Read the model definition and answer for the solid it produces. Units are mm, in the model's axes. Face numbers are marked on the shaded views. A direction names the side the tool comes from. Round coordinates to 2 decimals unless told otherwise and drop trailing zeros. Write each loop counter-clockwise with the first axis right and the second up, starting at its lowest first coordinate (ties: lowest second). Pieces come first, ordered by that corner, then holes. Notation, with made-up numbers: (79.5, 27) -> (99.5, 27) arc R8 cw to (99.5, 34) -> close; hole circle Ø6 at (88, 46.25). An arc over 180 degrees is marked (long way). Return JSON: item names as keys, results as strings.
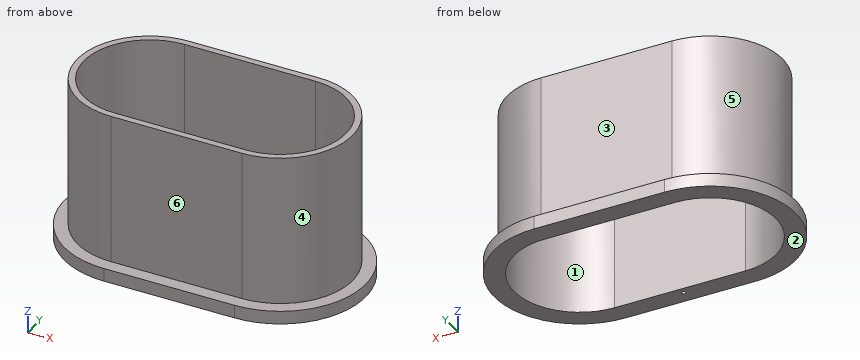
from build123d import *

# Parameters (mm, degrees)
EXTRUDE_1_DEPTH     = 2
EXTRUDE_2_DEPTH     = 23
SKETCH_4_R          = 0.3
CUT_EXTRUDE_2_DEPTH = 0.5


with BuildPart() as part:
    # 草图1 → 凸台-拉伸1 (new body)
    with BuildSketch(Plane.XY):
        with BuildLine():
            Line((-7.168044136, -16.461643491), (-27.168044136, -16.461643491))
            ThreePointArc((-27.168044136, -16.461643491), (-40.168044136, -3.461643491), (-27.168044136, 9.538356509))
            Line((-27.168044136, 9.538356509), (-7.168044136, 9.538356509))
            ThreePointArc((-7.168044136, 9.538356509), (5.831955864, -3.461643491), (-7.168044136, -16.461643491))
        make_face()
        with BuildLine():
            Line((-27.168044136, -13.461643491), (-7.168044136, -13.461643491))
            ThreePointArc((-7.168044136, -13.461643491), (2.831955864, -3.461643491), (-7.168044136, 6.538356509))
            Line((-7.168044136, 6.538356509), (-27.168044136, 6.538356509))
            ThreePointArc((-27.168044136, 6.538356509), (-37.168044136, -3.461643491), (-27.168044136, -13.461643491))
        make_face(mode=Mode.SUBTRACT)
    extrude(amount=EXTRUDE_1_DEPTH)

    # 草图2 → 凸台-拉伸2 (add)
    with BuildSketch(Plane.XY.offset(2)):
        with BuildLine():
            Line((-27.168044136, 7.538356509), (-7.168044136, 7.538356509))
            ThreePointArc((-7.168044136, 7.538356509), (3.831955864, -3.461643491), (-7.168044136, -14.461643491))
            Line((-7.168044136, -14.461643491), (-27.168044136, -14.461643491))
            ThreePointArc((-27.168044136, -14.461643491), (-38.168044136, -3.461643491), (-27.168044136, 7.538356509))
        make_face()
        with BuildLine():
            Line((-27.168044136, 6.538356509), (-7.168044136, 6.538356509))
            ThreePointArc((-7.168044136, 6.538356509), (2.831955864, -3.461643491), (-7.168044136, -13.461643491))
            Line((-7.168044136, -13.461643491), (-27.168044136, -13.461643491))
            ThreePointArc((-27.168044136, -13.461643491), (-37.168044136, -3.461643491), (-27.168044136, 6.538356509))
        make_face(mode=Mode.SUBTRACT)
    extrude(amount=EXTRUDE_2_DEPTH)

    # 草图4 → 切除-拉伸2 (cut)
    with BuildSketch(Plane(origin=(0, 0, 0), x_dir=(-1, 0, 0), z_dir=(0, 0, -1))):
        with Locations((17.168044136, -14.461643491)):
            Circle(SKETCH_4_R)
    extrude(amount=-CUT_EXTRUDE_2_DEPTH, mode=Mode.SUBTRACT)


solid = part.part
Item 1: Section A-A (x = -23.5) is taken. Give the vertices of the cut face in (y, z).
Worked answers:
{"outline": "(-16.46, 0) -> (-13.46, 0) -> (-13.46, 25) -> (-14.46, 25) -> (-14.46, 2) -> (-16.46, 2) -> close; (6.54, 0) -> (9.54, 0) -> (9.54, 2) -> (7.54, 2) -> (7.54, 25) -> (6.54, 25) -> close"}
Item 2: For a pull along Y with two mould halves and no side action, classify the marked faces 1, 2 and 3 as released by +Y, released by -Y, zero draft, split by the parting line, or undercut.
Worked answers:
{"face 1": "undercut", "face 2": "zero draft", "face 3": "released by +Y"}
Item 3: Flat-ended cylindrical pins translate along their axes: pin 1 (4 mm diameter, centred on x = -16.5, z = 18, fed in from +Y); pin 2 (1 mm diameter, centred on x = 0, z = 10, fed in from +Y); pin 3 (12 mm diameter, centred on y = -5, z = 21.5, fed in from +X); pin 4 (1 mm diameter, centred on x = -35.5, y = 5, fed in from -Z). Find the tip coordinate at first contact, or state that the pin passes through.
Worked answers:
{"pin 1": "stops at y = 7.54", "pin 2": "stops at y = 5.29", "pin 3": "stops at x = 3.83", "pin 4": "stops at z = 0"}
Item 4: Straight lines are drawn through the part: L1, parallel to Y at x = -17, z = 14.75; L2, parallel to Z at x = -9.5, y = 8.25; L3, parallel to Y at x = 2, z = 12 (3 decimals). For each, find the intervals that lie inside material, in ascending order. Write a range as [from, to].
Worked answers:
{"L1": "y = [-14.46, -13.46], [6.54, 7.54]", "L2": "z = [0, 2]", "L3": "y = [-9.54, -7.455], [0.532, 2.617]"}
Item 5: A tool of negligible diameter and unlimited length cuts with its end or side. For the marked faces 4, 5 and 6, from which of +Z, -Z, +X, -X, +Y, -Y can it reach the whole face along a straight path? Write none if from no direction.
Worked answers:
{"face 4": "+Z, +X", "face 5": "+Z, -X", "face 6": "+Z, +X, -X, -Y"}
Item 6: Section B-B (z = 8.25) is taken. Give the vertices of the cut face in (x, y), then the cut area to 3 significant figures.
Worked answers:
{"outline": "(-27.17, -14.46) -> (-7.17, -14.46) arc R11 ccw to (-7.17, 7.54) -> (-27.17, 7.54) arc R11 ccw to start; hole (-27.17, -13.46) -> (-7.17, -13.46) arc R10 ccw to (-7.17, 6.54) -> (-27.17, 6.54) arc R10 ccw to start", "area": "106 mm2"}
Item 7: Section C-C (y = -0.5) is taken. Give the vertices of the cut face in (x, z).
Worked answers:
{"outline": "(-39.83, 0) -> (-36.72, 0) -> (-36.72, 25) -> (-37.76, 25) -> (-37.76, 2) -> (-39.83, 2) -> close; (2.38, 0) -> (5.49, 0) -> (5.49, 2) -> (3.43, 2) -> (3.43, 25) -> (2.38, 25) -> close"}
